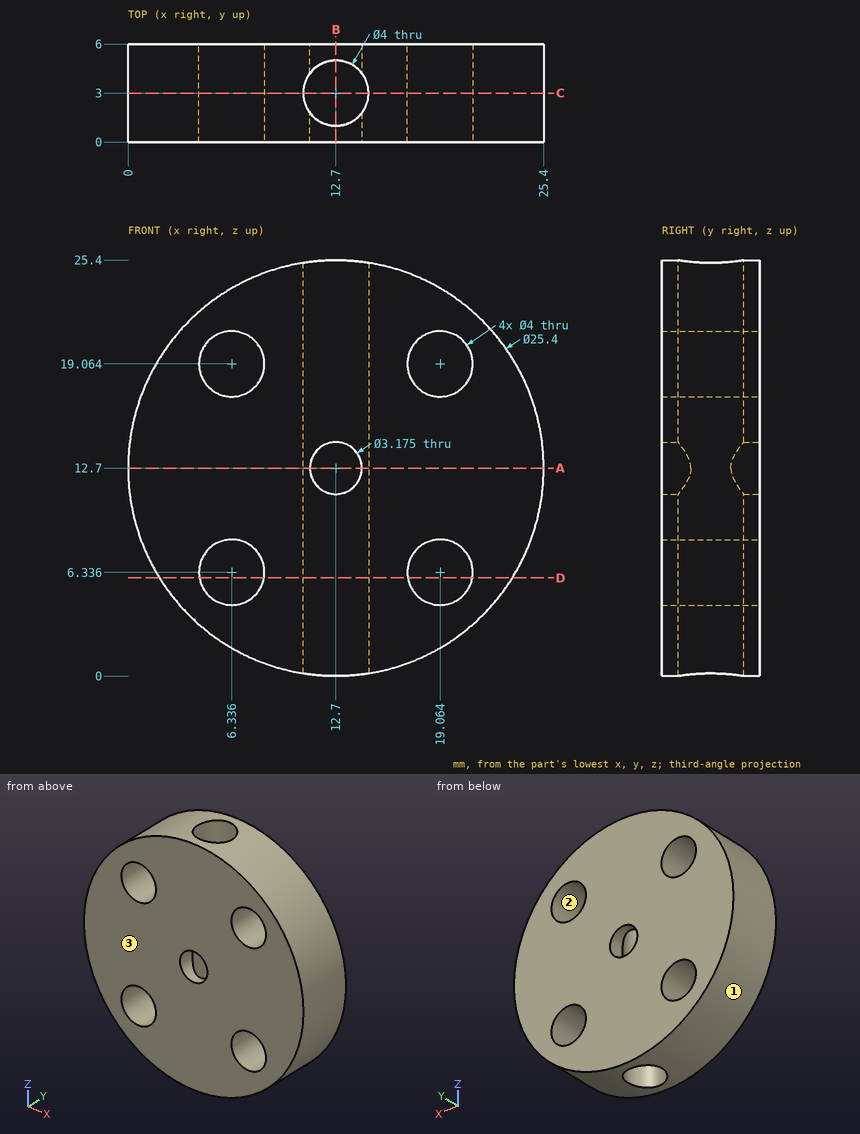
Part print with two shaded views. Sizes in mm from the minimum x, y, z corner. Coordinates: 2 decimals unless noted, no trailing zeros. Write each loop counter-clockwise with the first axis right and the second up, starting at its lowest first coordinate (ties: lowest second). Pieces come first, ordered by that corner, then holes. Notation, with made-up numbers: (44.5, -35.5) - (80.5, -35.5) arc R13 ccw to (80.5, -13.5) - close; hole circle Ø9 at (75.25, -4). An arc over 180 degrees is marked (long way). One line per item, written item: value. Start each with the question number.
1. Flat gauge pins, fed straight in: pin 1 (3.5 mm diameter, centred on x = 12.7, y = 3, fed in from +Z); pin 2 (3 mm diameter, centred on x = 15, y = 1.5, fed in from -Z). Where does each tip first touch, or does it go through?
2. Slice it at A-A (z = 12.7). Write the cut outline in (x, y), plus the area to 3 significant figures.
3. Slice it at B-B (x = 12.7). Write the cut outline in (y, z).
4. Probe line 1 (X direction, y = 0.5, z = 7.75); line 2 (Y direction, x = 12.7, z = 5); line 3 (X direction, y = 0.75, z = 17.25). List the from-to ranges inside material, lowest first. Write a range as from..to.
5. Mould opens along Z. For the marked faces 1, 2 and 3 say: released by +Z, released by -Z, zero draft, split by the parting line, or undercut.
6. Slice it at C-C (y = 3). Write the cut outline in (x, z), plus the area to 3 significant figures.
7. Slice it at D-D (z = 6). Write the cut outline in (x, y), plus the area to 3 significant figures.
Answers below:
1. pin 1: passes through
1. pin 2: stops at z = 0.03
2. outline: (0, 0) - (11.11, 0) - (11.11, 1.78) arc R2 cw to (11.11, 4.22) - (11.11, 6) - (0, 6) - close; (14.29, 0) - (25.4, 0) - (25.4, 6) - (14.29, 6) - (14.29, 4.22) arc R2 cw to (14.29, 1.78) - close
2. area: 132 mm^2
3. outline: (0, 0) - (1, 0) - (1, 11.11) - (0, 11.11) - close; (0, 14.29) - (1, 14.29) - (1, 25.4) - (0, 25.4) - close; (5, 0) - (6, 0) - (6, 11.11) - (5, 11.11) - close; (5, 14.29) - (6, 14.29) - (6, 25.4) - (5, 25.4) - close
4. line 1: x = 1..4.92, 7.75..17.65, 20.48..24.4
4. line 2: y = 0..1, 5..6
4. line 3: x = 0.84..5.49, 7.18..18.22, 19.91..24.56
5. face 1: split by the parting line
5. face 2: undercut
5. face 3: zero draft
6. outline: (10.7, 0.16) - (10.7, 25.24) arc R12.7 ccw to start; (14.7, 0.16) arc R12.7 ccw to (14.7, 25.24) - close; hole circle Ø4 at (6.34, 6.34); hole circle Ø4 at (6.34, 19.06); hole circle Ø4 at (19.06, 6.34); hole circle Ø4 at (19.06, 19.06)
6. area: 355 mm^2
7. outline: (1.91, 0) - (4.36, 0) - (4.36, 6) - (1.91, 6) - close; (8.31, 0) - (17.09, 0) - (17.09, 6) - (8.31, 6) - close; (21.04, 0) - (23.49, 0) - (23.49, 6) - (21.04, 6) - close; hole circle Ø4 at (12.7, 3)
7. area: 69.6 mm^2
